```python
from build123d import *

# Parameters (mm, degrees)
SKETCH1_W                  = 44.45
SKETCH1_H                  = 25.4
BOSS_EXTRUDE1_DEPTH        = 9.525
CHAMFER1_SIZE              = 6.35
HOLE1_AT_2_COUNT           = 2
HOLE1_AT_2_PITCH           = 30.13075
F_8_0_199_DIAMETER_HOLE1_D = 5.0546
CHAMFER2_SIZE              = 0.762


with BuildPart() as part:
    # Sketch1 → Boss-Extrude1 (new body)
    with BuildSketch(Plane.XY):
        with Locations((35.268404938, -193.371995598)):
            Rectangle(SKETCH1_W, SKETCH1_H)
        Polygon((43.174154938, -197.936382488), (43.174154938, -188.807608707), (35.268404938, -184.243221816), (27.362654938, -188.807608707), (27.362654938, -197.936382488), (35.268404938, -202.500769379), align=None, mode=Mode.SUBTRACT)
    extrude(amount=BOSS_EXTRUDE1_DEPTH)

    # Chamfer1
    chamfer1_edges = [part.edges().sort_by_distance(p)[0] for p in [
        (13.043404938, -180.671995598, 4.7625),
        (57.493404938, -180.671995598, 4.7625),
        (57.493404938, -206.071995598, 4.7625),
        (13.043404938, -206.071995598, 4.7625),
    ]]
    chamfer(chamfer1_edges, length=CHAMFER1_SIZE)

    # Sketch3 → Hole1 (revolve, cut)
    with BuildSketch(Plane(origin=(20.203029938, -193.371995598, 0), x_dir=(0, 1, 0), z_dir=(1, 0, 0))):
        Polygon((0, 0), (0, 4.699), (2.8702, 4.699), (2.9972, 0), align=None)
    hole1 = revolve(axis=Axis((20.203029938, -193.371995598, 110), (0, 0, -1)), mode=Mode.SUBTRACT)

    # Hole1 at 2: Hole1 ×2
    with Locations(*[(i * HOLE1_AT_2_PITCH, 0, 0) for i in range(1, HOLE1_AT_2_COUNT)]):
        add(hole1, mode=Mode.SUBTRACT)

    # #8 (0.199) Diameter Hole1 (through all)
    with Locations(Plane(origin=(0, 0, 0), x_dir=(-1, 0, 0), z_dir=(0, 0, -1))):
        with Locations((-50.333779938, -193.371995598), (-20.203029938, -193.371995598)):
            Hole(F_8_0_199_DIAMETER_HOLE1_D / 2)

    # Chamfer2
    chamfer2_edges = [part.edges().sort_by_distance(p)[0] for p in [
        (39.221279938, -200.218575934, 0),
        (43.174154938, -193.371995598, 0),
        (39.221279938, -186.525415262, 0),
        (31.315529938, -186.525415262, 0),
        (27.362654938, -193.371995598, 0),
        (31.315529938, -200.218575934, 0),
        (39.221279938, -200.218575934, 9.525),
        (43.174154938, -193.371995598, 9.525),
        (39.221279938, -186.525415262, 9.525),
        (31.315529938, -186.525415262, 9.525),
        (27.362654938, -193.371995598, 9.525),
        (31.315529938, -200.218575934, 9.525),
        (35.268404938, -180.671995598, 0),
        (35.268404938, -180.671995598, 9.525),
        (13.043404938, -193.371995598, 0),
        (57.493404938, -193.371995598, 0),
        (35.268404938, -206.071995598, 0),
        (16.218404938, -183.846995598, 0),
        (16.218404938, -202.896995598, 0),
        (54.318404938, -202.896995598, 0),
        (54.318404938, -183.846995598, 0),
        (57.493404938, -193.371995598, 9.525),
        (13.043404938, -193.371995598, 9.525),
        (35.268404938, -206.071995598, 9.525),
        (16.218404938, -183.846995598, 9.525),
        (16.218404938, -202.896995598, 9.525),
        (54.318404938, -202.896995598, 9.525),
        (54.318404938, -183.846995598, 9.525),
        (17.675729938, -193.371995598, 9.525),
        (47.806479938, -193.371995598, 9.525),
    ]]
    chamfer(chamfer2_edges, length=CHAMFER2_SIZE)


solid = part.part
```
Build history of the part. All positions in model axes, mm. A direction names the side the tool comes from. Give positions to 0.01 mm unless a question says otherwise; leave off trailing zeros. Loops run counter-clockwise (first coordinate to the right, second up) from the corner with the lowest first, then second, coordinate; pieces in that order, holes last. Notation, with made-up numbers: (58, 45) -> (112, 45) arc R28 ccw to (112, 70) -> close; hole circle Ø6 at (67.25, 73). An arc over 180 degrees is marked (long way). One line per question, with ' | ' between items.
Q1. Drill centre lines: line 1 along X through (y, z) = (-192.75, 1); line 2 along Y through (x, z) = (20, 8.75); line 3 along X through (y, z) = (-195.75, 1.5). Where is each one in solid material? Low to high. Write a range as [from, to].
Filled sheet:
line 1: x = [13.04, 17.3], [23.11, 27.36], [43.17, 47.43], [53.24, 57.49] | line 2: y = [-206.07, -195.89], [-190.85, -180.67] | line 3: x = [13.04, 18.45], [21.96, 27.36], [43.17, 48.58], [52.09, 57.49]
Q2. Drop flat-ended pins along their axis: pin 1 (1.7 mm diameter, centred on x = 20, y = -192, fed in from -Z); pin 2 (2 mm diameter, centred on x = 18, z = 8, fed in from +Y). Give the stop position or say it passes through.
Filled sheet:
pin 1: passes through | pin 2: stops at y = -181.07
Q3. Tool access for faces 1 (the flat face through (31.371, -186.493, 4.706)), 2 (the flat face through (39.47, -186.24, 0.39)), 3 (the flat face through (54.36, -183.89, 4.71)), 4 (the flat face through (31.07, -200.51, 9.14)): list every direction of +Z, -Z, +X, -X, +Y, -Y with a clear straight run to the whole face (end or side of a thin tool).
Filled sheet:
face 1: +Z, -Z | face 2: -Z | face 3: +Z, -Z, +X, +Y | face 4: +Z
Q4. Cut at B-B, the plane z = 6.5. Write the cut outline in (x, y), plus the area to 3 significant figures.
Filled sheet:
outline: (13.04, -199.72) -> (19.39, -206.07) -> (51.14, -206.07) -> (57.49, -199.72) -> (57.49, -187.02) -> (51.14, -180.67) -> (19.39, -180.67) -> (13.04, -187.02) -> close; hole circle Ø5.05 at (20.2, -193.37); hole (27.36, -197.94) -> (35.27, -202.5) -> (43.17, -197.94) -> (43.17, -188.81) -> (35.27, -184.24) -> (27.36, -188.81) -> close; hole circle Ø5.05 at (50.33, -193.37) | area: 792 mm²
Q5. Cut at C-C, the plane y = -201.5. Write the cut outline in (x, z) (3 decimals).
Filled sheet:
outline: (14.821, 0.762) -> (15.899, 0) -> (32.011, 0) -> (33.535, 0.762) -> (33.535, 8.763) -> (32.011, 9.525) -> (15.899, 9.525) -> (14.821, 8.763) -> close; (37.002, 0.762) -> (38.526, 0) -> (54.638, 0) -> (55.715, 0.762) -> (55.715, 8.763) -> (54.638, 9.525) -> (38.526, 9.525) -> (37.002, 8.763) -> close
Q6. Pull direction Y, two halves, no side cores. Call faces 5 (the flat face through (16.45, -184.16, 9.15)), 6 (the flat face through (31.19, -186.17, 0.39)), 7 (the flat face through (16.44, -202.59, 0.39)), 8 (the flat face through (13.043, -193, 5)): pulls with the +Y half, pulls with the -Y half, needs draft (parallel to the pull), parting line crosses it, or undercut.
Filled sheet:
face 5: pulls with the +Y half | face 6: undercut | face 7: pulls with the -Y half | face 8: needs draft
Q7. Cut at D-D, the plane x = 55.5. Write the cut outline in (y, z) (3 decimals).
Filled sheet:
outline: (-201.715, 0.762) -> (-200.638, 0) -> (-186.106, 0) -> (-185.029, 0.762) -> (-185.029, 8.763) -> (-186.106, 9.525) -> (-200.638, 9.525) -> (-201.715, 8.763) -> close
Q8. Cut at A-A, the plane x = 28. Write the cut outline in (y, z) (3 decimals), plus the area to 3 significant figures.
Filled sheet:
outline: (-206.072, 0.762) -> (-205.31, 0) -> (-199.184, 0) -> (-198.304, 0.762) -> (-198.304, 8.763) -> (-199.184, 9.525) -> (-205.31, 9.525) -> (-206.072, 8.763) -> close; (-188.44, 0.762) -> (-187.56, 0) -> (-181.434, 0) -> (-180.672, 0.762) -> (-180.672, 8.763) -> (-181.434, 9.525) -> (-187.56, 9.525) -> (-188.44, 8.763) -> close | area: 145 mm²
